from build123d import *

# Parameters (mm, degrees)
F0_R      = 25
F1_DEPTH  = 70
F2_R      = 7.5
F3_DEPTH  = 5
F4_R      = 5.975
F5_DEPTH  = 50
F6_DEPTH  = 70
F7_R      = 7.5
F8_DEPTH  = 5
F9_R      = 4.975
F10_DEPTH = 15


with BuildPart() as f1:
    # F0 (on Right) → F1 (new body)
    with BuildSketch(Plane.YZ):
        Circle(F0_R)
    extrude(amount=F1_DEPTH)

    # F2 (on face) → F3 (join)
    with BuildSketch(Plane.YZ.offset(70)):
        Circle(F2_R)
    extrude(amount=F3_DEPTH)

    # F4 (on face) → F5 (join)
    with BuildSketch(Plane.YZ.offset(75)):
        Circle(F4_R)
    extrude(amount=F5_DEPTH)

    # F6 (add): a face of the model
    f6_faces = [f1.faces().sort_by_distance(p)[0] for p in [
        (0, 0, 0),
    ]]
    extrude(f6_faces, amount=F6_DEPTH)

    # F7 (on face) → F8 (join)
    with BuildSketch(Plane(origin=(-70, 0, 0), x_dir=(0, -1, 0), z_dir=(-1, 0, 0))):
        Circle(F7_R)
    extrude(amount=F8_DEPTH)

    # F9 (on face) → F10 (join)
    with BuildSketch(Plane(origin=(-75, 0, 0), x_dir=(0, -1, 0), z_dir=(-1, 0, 0))):
        Circle(F9_R)
    extrude(amount=F10_DEPTH)


solid = f1.part
The model under review builds one solid part; all positions refer to its coordinate system, in mm. A direction names the side the tool comes from. Coordinates: 2 decimals unless noted, no trailing zeros. Write each loop counter-clockwise with the first axis right and the second up, starting at its lowest first coordinate (ties: lowest second). Pieces come first, ordered by that corner, then holes. Notation, with made-up numbers: M 4.25,73.5 L 37.25,73.5 A24 ccw 37.25,104.5 Z; hole C 1,33.25 d10. An arc over 180 degrees is marked long. Put each result on its own line as item: value.
1) Clearance check with flat-ended pins moving along their axes: pin 1 Ø12 at (x, z) = (95, 6) entering from +Y (3 decimals); pin 2 Ø6 at (y, z) = (14.5, -5.5) entering from -X; pin 3 Ø3 at (x, z) = (97.5, 4) entering from -Y. State where each tip first meets the part, or that it passes through.
Computed:
pin 1: stops at y = 5.975
pin 2: stops at x = -70
pin 3: stops at y = -5.43
2) Add section A-A on y = 0. Give the boundary of the cut face in (x, z) (3 decimals), then the cut area to 3 significant figures.
Computed:
outline: M -90,-4.975 L -75,-4.975 L -75,-7.5 L -70,-7.5 L -70,-25 L 70,-25 L 70,-7.5 L 75,-7.5 L 75,-5.975 L 125,-5.975 L 125,5.975 L 75,5.975 L 75,7.5 L 70,7.5 L 70,25 L -70,25 L -70,7.5 L -75,7.5 L -75,4.975 L -90,4.975 Z
area: 7,900 mm2
3) Add section D-D on x = 4.5. Give the boundary of the cut face in (y, z).
Computed:
outline: C 0,0 d50
4) For faces 1 (the flat face through (-90, 0, 0)), 2 (the flat face through (70, -6, -5)), 3 (the flat face through (-75, -2, -5)), list the 3-axis set-ups (+Z, -Z, +X, -X, +Y, -Y) from which the entire face can be reached by the end or side of a thin tool; tool diameter is ignored.
Computed:
face 1: +Z, -Z, -X, +Y, -Y
face 2: +X
face 3: -X
5) Add section C-C on x = 81. Give the boundary of the cut face in (y, z) (3 decimals), then the cut area to 3 significant figures.
Computed:
outline: C 0,0 d11.95
area: 112 mm2
6) Wall thickness on probe 1 along X at (y, z) = (-5.5, 8.5); probe 2 along Y at (x, z) = (-65.5, -1.5); probe 3 along Y at (x, z) = (61.5, 20): over which ranges is each line inside the solid? List them lowest first. Write a range as [from, to].
Computed:
probe 1: x = [-70, 70]
probe 2: y = [-24.95, 24.95]
probe 3: y = [-15, 15]
